CAD build for the part. Positions are in the model's coordinates, mm. Face numbers are marked on the shaded views. A direction names the side the tool comes from. Round coordinates to 2 decimals unless told otherwise and drop trailing zeros. Order: outer loops, then holes, each group sorted by start corner. A loop starts at its lowest first (then second) coordinate and runs counter-clockwise, first axis right, second up. Notation, with made-up numbers: M -13.5,48.25 L 28.5,48.25 A15 cw 28.5,71.25 Z; hole C 89,54.25 d10. An arc over 180 degrees is marked long. Answer as a JSON object with one key per item and string values. Group by question number.
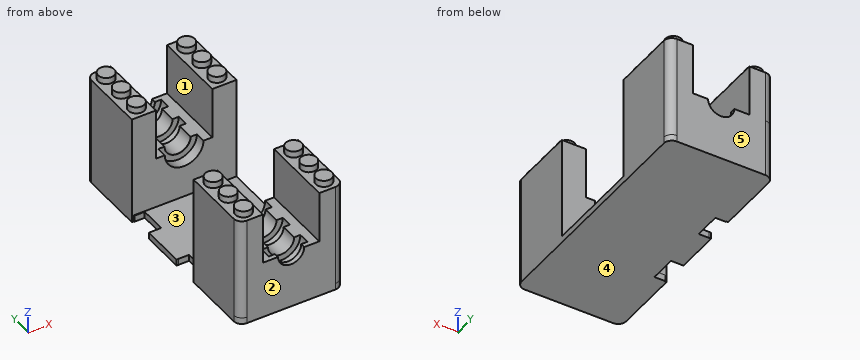
```python
from build123d import *

# Parameters (mm, degrees)
SKETCH1_W                 = 32.5
SKETCH1_H                 = 22.5
BOSS_EXTRUDE1_DEPTH       = 16
SKETCH2_W                 = 32.5
SKETCH2_H                 = 37.845937441
BOSS_EXTRUDE2_DEPTH       = 2
CUT_EXTRUDE2_DEPTH        = 59.458857784
SKETCH3_R                 = 6
SKETCH3_R_2               = 4.0625
CUT_EXTRUDE1_DEPTH        = 3.5
LPATTERN1_COUNT           = 3
LPATTERN1_PITCH           = 8.75
MIRROR7_COPY_1_SKETCH_R   = 6
MIRROR7_COPY_1_SKETCH_R_2 = 4.0625
MIRROR7_COPY_1_DEPTH      = 3.5
MIRROR7_COPY_2_SKETCH_R   = 6
MIRROR7_COPY_2_SKETCH_R_2 = 4.0625
MIRROR7_COPY_2_DEPTH      = 3.5
MIRROR7_COPY_3_SKETCH_R   = 6
MIRROR7_COPY_3_SKETCH_R_2 = 4.0625
MIRROR7_COPY_3_DEPTH      = 3.5
SKETCH5_W                 = 7.5
SKETCH5_H                 = 22.5
BOSS_EXTRUDE6_DEPTH       = 16
SKETCH6_R                 = 2.5
BOSS_EXTRUDE7_DEPTH       = 2
SKETCH7_W                 = 3.25
SKETCH7_H                 = 8.25
CUT_EXTRUDE3_DEPTH        = 10
LPATTERN2_COUNT           = 2
LPATTERN2_PITCH           = 7.5
LPATTERN3_COUNT           = 2
LPATTERN3_PITCH           = 7.5
BOSS_EXTRUDE8_START       = -18.845937441
BOSS_EXTRUDE8_DEPTH       = 0.25
BOSS_EXTRUDE9_START       = 18.595937441
BOSS_EXTRUDE9_DEPTH       = 0.25
FILLET1_R                 = 2.5
SKETCH10_W                = 0.625
SKETCH10_H                = 8.470937441
CUT_EXTRUDE4_DEPTH        = 54.407653766


# Read off the part's stored shape, not the designer's step: Boss-Extrude8, Boss-Extrude9
with BuildPart() as part:
    # Sketch1 → Boss-Extrude1 (new body)
    with BuildSketch(Plane.XY):
        with Locations((0, -26.595937441)):
            Rectangle(SKETCH1_W, SKETCH1_H)
    boss_extrude1 = extrude(amount=-BOSS_EXTRUDE1_DEPTH)

    # Sketch2 → Boss-Extrude2 (add)
    with BuildSketch(Plane(origin=(0, 0, -16), x_dir=(-1, 0, 0), z_dir=(0, 0, -1))):
        with Locations((0, -18.922968721)):
            Rectangle(SKETCH2_W, SKETCH2_H)
    boss_extrude2 = extrude(amount=BOSS_EXTRUDE2_DEPTH)

    # Mirror4: Boss-Extrude2 across plane
    add(boss_extrude2.mirror(Plane(origin=(-16.25, 0, -18), x_dir=(0, 0, 1), z_dir=(0, -1, 0))))

    # Mirror5: Boss-Extrude1 across plane
    add(boss_extrude1.mirror(Plane.ZX))

    # Sketch3<3> → Cut-Extrude2 (cut, through all)
    with BuildSketch(Plane(origin=(0, -15.345937441, 0), x_dir=(1, 0, 0), z_dir=(0, 1, 0))):
        with BuildLine():
            Line((-4.0625, 0), (4.0625, 0))
            ThreePointArc((4.0625, 0), (0, 4.0625), (-4.0625, 0))
        make_face()
        with BuildLine():
            ThreePointArc((-4.0625, 0), (0, -4.0625), (4.0625, 0))
            Line((4.0625, 0), (-4.0625, 0))
        make_face()
    cut_extrude2 = extrude(amount=-CUT_EXTRUDE2_DEPTH, mode=Mode.SUBTRACT)

    # Sketch3 → Cut-Extrude1 (cut)
    with BuildSketch(Plane(origin=(0, -15.345937441, 0), x_dir=(1, 0, 0), z_dir=(0, 1, 0))):
        Circle(SKETCH3_R)
        Circle(SKETCH3_R_2, mode=Mode.SUBTRACT)
    cut_extrude1 = extrude(amount=-CUT_EXTRUDE1_DEPTH, mode=Mode.SUBTRACT)

    # LPattern1: Cut-Extrude1 ×3
    with Locations(*[(0, -i * LPATTERN1_PITCH, 0) for i in range(1, LPATTERN1_COUNT)]):
        add(cut_extrude1, mode=Mode.SUBTRACT)

    # Mirror6: Cut-Extrude2, Cut-Extrude1 across plane
    add(cut_extrude2.mirror(Plane.ZX), mode=Mode.SUBTRACT)
    add(cut_extrude1.mirror(Plane.ZX), mode=Mode.SUBTRACT)

    # Mirror6 at the second plane: Cut-Extrude2, Cut-Extrude1 across plane
    add(cut_extrude2.mirror(Plane.XY), mode=Mode.SUBTRACT)
    add(cut_extrude1.mirror(Plane.XY), mode=Mode.SUBTRACT)

    # Mirror7 copy 1 sketch → Mirror7 copy 1 (cut)
    with BuildSketch(Plane.XZ.offset(-24.095937441)):
        Circle(MIRROR7_COPY_1_SKETCH_R)
        Circle(MIRROR7_COPY_1_SKETCH_R_2, mode=Mode.SUBTRACT)
    extrude(amount=-MIRROR7_COPY_1_DEPTH, mode=Mode.SUBTRACT)

    # Mirror7 copy 2 sketch → Mirror7 copy 2 (cut)
    with BuildSketch(Plane.XZ.offset(-32.845937441)):
        Circle(MIRROR7_COPY_2_SKETCH_R)
        Circle(MIRROR7_COPY_2_SKETCH_R_2, mode=Mode.SUBTRACT)
    extrude(amount=-MIRROR7_COPY_2_DEPTH, mode=Mode.SUBTRACT)

    # Mirror7 copy 3 sketch → Mirror7 copy 3 (cut)
    with BuildSketch(Plane.XZ.offset(-15.345937441)):
        Circle(MIRROR7_COPY_3_SKETCH_R)
        Circle(MIRROR7_COPY_3_SKETCH_R_2, mode=Mode.SUBTRACT)
    extrude(amount=-MIRROR7_COPY_3_DEPTH, mode=Mode.SUBTRACT)

    # Sketch5 → Boss-Extrude6 (add)
    with BuildSketch(Plane.XY):
        with Locations((-12.5, -26.595937441)):
            Rectangle(SKETCH5_W, SKETCH5_H)
        with Locations((12.5, -26.595937441)):
            Rectangle(SKETCH5_W, SKETCH5_H)
        with Locations((12.5, 26.595937441)):
            Rectangle(SKETCH5_W, SKETCH5_H)
        with Locations((-12.5, 26.595937441)):
            Rectangle(SKETCH5_W, SKETCH5_H)
    extrude(amount=BOSS_EXTRUDE6_DEPTH)

    # Sketch6 → Boss-Extrude7 (add)
    with BuildSketch(Plane.XY.offset(16)):
        with Locations(Location((-12.5, -26.595937441, 0), (0, 0, 180))):
            Circle(SKETCH6_R)
        with Locations(Location((-12.5, 26.595937441, 0), (0, 0, 180))):
            Circle(SKETCH6_R)
        with Locations((12.5, 26.595937441)):
            Circle(SKETCH6_R)
        with Locations(Location((12.5, -26.595937441, 0), (0, 0, 180))):
            Circle(SKETCH6_R)
    boss_extrude7 = extrude(amount=BOSS_EXTRUDE7_DEPTH)

    # Sketch7 → Cut-Extrude3 (cut)
    with BuildSketch(Plane(origin=(0, 0, -18), x_dir=(-1, 0, 0), z_dir=(0, 0, -1))):
        with Locations((14, -11)):
            Rectangle(SKETCH7_W, SKETCH7_H)
        with Locations((14, 11)):
            Rectangle(SKETCH7_W, SKETCH7_H)
    extrude(amount=-CUT_EXTRUDE3_DEPTH, mode=Mode.SUBTRACT)

    # LPattern2: Boss-Extrude7 ×2
    with Locations(*[(0, -i * LPATTERN2_PITCH, 0) for i in range(1, LPATTERN2_COUNT)]):
        add(boss_extrude7)

    # LPattern3: Boss-Extrude7 ×2
    with Locations(*[(0, i * LPATTERN3_PITCH, 0) for i in range(1, LPATTERN3_COUNT)]):
        add(boss_extrude7)

    # Boss-Extrude8 outline → Boss-Extrude8 (add)
    with BuildSketch(Plane(origin=(0, 0, 0), x_dir=(1, 0, 0), z_dir=(0, 1, 0)).offset(BOSS_EXTRUDE8_START)):
        with BuildLine():
            ThreePointArc((-4.0625, 0), (0, 4.0625), (4.0625, 0))
            Line((4.0625, 0), (6, 0))
            ThreePointArc((6, 0), (0, 6), (-6, 0))
            Line((-6, 0), (-4.0625, 0))
        make_face()
    extrude(amount=BOSS_EXTRUDE8_DEPTH)

    # Boss-Extrude9 outline → Boss-Extrude9 (add)
    with BuildSketch(Plane(origin=(0, 0, 0), x_dir=(1, 0, 0), z_dir=(0, 1, 0)).offset(BOSS_EXTRUDE9_START)):
        with BuildLine():
            ThreePointArc((6, 0), (0, 6), (-6, 0))
            Line((-6, 0), (-4.0625, 0))
            ThreePointArc((-4.0625, 0), (0, 4.0625), (4.0625, 0))
            Line((4.0625, 0), (6, 0))
        make_face()
    extrude(amount=BOSS_EXTRUDE9_DEPTH)

    # Fillet1
    fillet1_edges = [part.edges().sort_by_distance(p)[0] for p in [
        (-16.25, 37.845937441, -1),
        (16.25, 37.845937441, -1),
        (16.25, -37.845937441, -1),
        (-16.25, -37.845937441, -1),
    ]]
    fillet(fillet1_edges, radius=FILLET1_R)

    # Sketch10 → Cut-Extrude4 (cut, through all)
    with BuildSketch(Plane.XY.offset(-16)):
        with Locations((-15.9375, 11.110468721)):
            Rectangle(SKETCH10_W, SKETCH10_H)
        with Locations((-15.9375, -11.110468721)):
            Rectangle(SKETCH10_W, SKETCH10_H)
    extrude(amount=-CUT_EXTRUDE4_DEPTH, mode=Mode.SUBTRACT)


solid = part.part
```
Item 1: 3-axis set-ups, long thin cutter, end or side, ignore diameter. For the marked faces 1 and 2: which of +Z, -Z, +X, -X, +Y, -Y reach the whole face in a straight line?
Item 2: Flat gauge pins, fed straight in: pin 1 Ø4 at (x, y) = (-5.5, 28.5) entering from +Z; pin 2 Ø0.6 at (y, z) = (12.5, -16.5) entering from -X (3 decimals); pin 3 Ø1 at (x, y) = (6.5, 6.5) entering from +Z. Where does each tip first touch, or does it go through?
Item 3: Cut at C-C, the plane y = -25. Give the cut face in (x, z), and give its area (3 significant figures).
Item 4: Cut at A-A, the plane z = 1. Give the cut face in (x, y).
Item 5: Cut at B-B, the plane x = 0. Give the cut face in (y, z), and give its area (3 significant figures).
Item 6: Two-plate mould, pull along Y, no slides. Class the marked faces 3, 4 and 5: +Y half, -Y half, draft (parallel to the pull), parting line (faces both ways), or undercut.
Item 7: Drill centre lines: line 1 (Y direction, x = 10, z = 15.5); line 2 (X direction, y = -21, z = 9.5); line 3 (Z direction, x = 5, y = -4.5). Where is each one in solid material? Low to high. Write a range as [from, to].
Response values:
{
 "1": {"face 1": "+Z, +Y, -Y", "face 2": "+Z, -Z, +X, -X, -Y"},
 "2": {"pin 1": "z = 0", "pin 2": "x = -12.375", "pin 3": "z = -16"},
 "3": {"outline": "M -16.25,-18 L 16.25,-18 L 16.25,16 L 14.42,16 L 14.42,18 L 10.58,18 L 10.58,16 L 8.75,16 L 8.75,0 L 6,0 A6 cw -6,0 L -8.75,0 L -8.75,16 L -10.58,16 L -10.58,18 L -14.42,18 L -14.42,16 L -16.25,16 Z", "area": "784 mm^2"},
 "4": {"outline": "M -16.25,-35.35 A2.5 ccw -13.75,-37.85 L -8.75,-37.85 L -8.75,-15.35 L -16.25,-15.35 Z; M -16.25,15.35 L -8.75,15.35 L -8.75,37.85 L -13.75,37.85 A2.5 ccw -16.25,35.35 Z; M 8.75,-37.85 L 13.75,-37.85 A2.5 ccw 16.25,-35.35 L 16.25,-15.35 L 8.75,-15.35 Z; M 8.75,15.35 L 16.25,15.35 L 16.25,35.35 A2.5 ccw 13.75,37.85 L 8.75,37.85 Z"},
 "5": {"outline": "M -37.85,-18 L 37.85,-18 L 37.85,-4.06 L 36.35,-4.06 L 36.35,-6 L 32.85,-6 L 32.85,-4.06 L 27.6,-4.06 L 27.6,-6 L 24.1,-6 L 24.1,-4.06 L 18.6,-4.06 L 18.6,-6 L 15.35,-6 L 15.35,-16 L -15.35,-16 L -15.35,-6 L -18.6,-6 L -18.6,-4.06 L -24.1,-4.06 L -24.1,-6 L -27.6,-6 L -27.6,-4.06 L -32.85,-4.06 L -32.85,-6 L -36.35,-6 L -36.35,-4.06 L -37.85,-4.06 Z", "area": "649 mm^2"},
 "6": {"face 3": "undercut", "face 4": "draft", "face 5": "+Y half"},
 "7": {"line 1": "[-37.85, -15.35], [15.35, 37.85]", "line 2": "[-16.25, -8.75], [8.75, 16.25]", "line 3": "[-18, -16]"}
}
